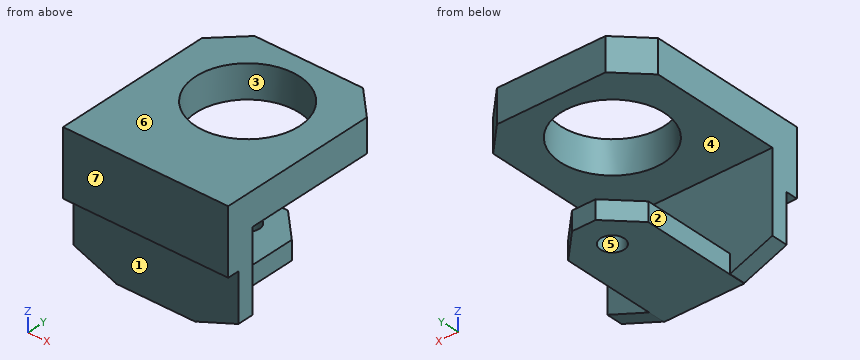
```python
from build123d import *

# Parameters (mm, degrees)
SKETCH1_W           = 35
SKETCH1_H           = 40
SKETCH1_R           = 11
BOSS_EXTRUDE1_DEPTH = 7
SKETCH2_W           = 35
SKETCH2_H           = 6
BOSS_EXTRUDE2_DEPTH = 16.5
SKETCH3_W           = 17
SKETCH3_H           = 32
SKETCH3_R           = 2.5
BOSS_EXTRUDE3_DEPTH = 4
CHAMFER1_SIZE       = 10.2
CHAMFER1_SIZE_2     = 3.915413157
CHAMFER2_SIZE       = 6
SKETCH4_W           = 35
SKETCH4_H           = 2.5
CUT_EXTRUDE1_DEPTH  = 13.7


with BuildPart() as part:
    # Sketch1 → Boss-Extrude1 (new body)
    with BuildSketch(Plane.XY):
        with Locations((0, -5)):
            Rectangle(SKETCH1_W, SKETCH1_H)
        Circle(SKETCH1_R, mode=Mode.SUBTRACT)
    extrude(amount=BOSS_EXTRUDE1_DEPTH)

    # Sketch2 → Boss-Extrude2 (add)
    with BuildSketch(Plane(origin=(0, 0, 0), x_dir=(-1, 0, 0), z_dir=(0, 0, -1))):
        with Locations((0, -22)):
            Rectangle(SKETCH2_W, SKETCH2_H)
    extrude(amount=BOSS_EXTRUDE2_DEPTH)

    # Sketch3 → Boss-Extrude3 (add)
    with BuildSketch(Plane(origin=(0, 0, -16.5), x_dir=(-1, 0, 0), z_dir=(0, 0, -1))):
        with Locations((0, -9)):
            Rectangle(SKETCH3_W, SKETCH3_H)
        Circle(SKETCH3_R, mode=Mode.SUBTRACT)
    extrude(amount=BOSS_EXTRUDE3_DEPTH)

    # Chamfer1
    # the kernel refuses this chamfer: 10.2, 3.915413157 mm, written as the material it adds along each edge
    with BuildSketch(Plane(origin=(-8.5, -19, -16.5), x_dir=(-0.9999045356599434, 0, 0.013817364679016049), z_dir=(0, -1, 0))) as chamfer1_piece_1_section:
        Polygon((CHAMFER1_SIZE * 0.99990453566, CHAMFER1_SIZE * 0.013817364679), (-CHAMFER1_SIZE_2 * 0.0138173646803, CHAMFER1_SIZE_2 * 0.999904535752), (0, 0), align=None)
    chamfer1_piece_1 = extrude(amount=6, mode=Mode.PRIVATE)
    chamfer1_piece_1 = split(chamfer1_piece_1, bisect_by=Plane(origin=(-17.5, -22, -17.821300415), z_dir=(1, 0, 0)), keep=Keep.TOP, mode=Mode.PRIVATE)
    add(chamfer1_piece_1)
    with BuildSketch(Plane(origin=(8.5, -25, -16.5), x_dir=(0.9999045356599434, 0, 0.013817364679016049), z_dir=(0, 1, 0))) as chamfer1_piece_2_section:
        Polygon((CHAMFER1_SIZE * 0.99990453566, CHAMFER1_SIZE * 0.013817364679), (-CHAMFER1_SIZE_2 * 0.0138173646803, CHAMFER1_SIZE_2 * 0.999904535752), (0, 0), align=None)
    chamfer1_piece_2 = extrude(amount=6, mode=Mode.PRIVATE)
    chamfer1_piece_2 = split(chamfer1_piece_2, bisect_by=Plane(origin=(17.5, -22, -17.821300415), z_dir=(-1, 0, 0)), keep=Keep.TOP, mode=Mode.PRIVATE)
    add(chamfer1_piece_2)

    # Chamfer2
    chamfer2_edges = [part.edges().sort_by_distance(p)[0] for p in [
        (-8.5, 7, -18.5),
        (8.5, 7, -18.5),
        (17.5, 15, 3.5),
        (-17.5, 15, 3.5),
    ]]
    chamfer(chamfer2_edges, length=CHAMFER2_SIZE)

    # Sketch4 → Cut-Extrude1 (cut)
    with BuildSketch(Plane(origin=(0, 0, -20.5), x_dir=(-1, 0, 0), z_dir=(0, 0, -1))):
        with Locations((0, -23.75)):
            Rectangle(SKETCH4_W, SKETCH4_H)
    extrude(amount=-CUT_EXTRUDE1_DEPTH, mode=Mode.SUBTRACT)


solid = part.part
```
Can you work these out from the model? Positions are in its coordinate system, mm. Face numbers are marked on the shaded views. A direction names the side the tool comes from. Give positions to 0.01 mm unless a question says otherwise; leave off trailing zeros. Loops run counter-clockwise (first coordinate to the right, second up) from the corner with the lowest first, then second, coordinate; pieces in that order, holes last. Notation, with made-up numbers: M 66,-25.75 L 111,-25.75 A33 ccw 111,9.25 Z; hole C -26.5,66.5 d5. An arc over 180 degrees is marked long. Use one line per item in the form item = value. Start each with the question number.
(1) I want a section at B-B, the plane y = -17.5. Write out the boundary of the cut face in (x, z), and give its area (3 significant figures).
(2) On a 3-axis mill with a long thin cutter (end or side, diameter ignored), from which of +Z, -Z, +X, -X, +Y, -Y can I reach the whole of each face in a straight line? I mean the marked faces 1, 2, 3 and 4. Say none if no direction works.
(3) I'm going to push flat-ended pins straight in: P1, Ø7, axis at x = -5.5, z = -14, coming from the -Y side; P2, Ø3, axis at x = -1.5, z = -16, coming from the +Y side; P3, Ø4.5, axis at y = -7, z = -18.5, coming from the -X side; P4, Ø1.5, axis at y = 0.5, z = -1.5, coming from the -X side. Where does each tip first touch, or does it pass through?
(4) Please list where these lines run through material, in increasing order: line 1 (Y direction, x = 0, z = 4); line 2 (Y direction, x = 0, z = -17.95); line 3 (Y direction, x = -4, z = -10.75).
(5) Thinking about a two-plate mould opening in Y: for the marked faces 5, 6 and 7, which applies, released by +Y, released by -Y, zero draft, split by the parting line, or undercut?
(6) I want a section at C-C, the plane y = 0. Write out the boundary of the cut face in (x, z).
(7) I want a section at D-D, the plane z = 5.25. Write out the boundary of the cut face in (x, y).
(8) I want a section at A-A, the plane x = 0. Write out the boundary of the cut face in (y, z).
Worked out:
q1.outline = M -17.5,0 L 17.5,0 L 17.5,7 L -17.5,7 Z; M -8.5,-20.5 L 8.5,-20.5 L 8.5,-16.5 L -8.5,-16.5 Z
q1.area = 313 mm²
q2.face_1 = -Z, +X, -X, -Y
q2.face_2 = -Z, -X, +Y
q2.face_3 = +Z
q2.face_4 = +X, -X, +Y
q3.P1 = -22.5
q3.P2 = 7
q3.P3 = -8.5
q3.P4 = through
q4.line_1 = -25 to -11, 11 to 15
q4.line_2 = -22.5 to -2.5, 2.5 to 7
q4.line_3 = -22.5 to -19
q5.face_5 = undercut
q5.face_6 = zero draft
q5.face_7 = released by -Y
q6.outline = M -17.5,0 L -11,0 L -11,7 L -17.5,7 Z; M -8.5,-20.5 L -2.5,-20.5 L -2.5,-16.5 L -8.5,-16.5 Z; M 2.5,-20.5 L 8.5,-20.5 L 8.5,-16.5 L 2.5,-16.5 Z; M 11,0 L 17.5,0 L 17.5,7 L 11,7 Z
q7.outline = M -17.5,-25 L 17.5,-25 L 17.5,9 L 11.5,15 L -11.5,15 L -17.5,9 Z; hole C 0,0 d22
q8.outline = M -25,-6.8 L -22.5,-6.8 L -22.5,-20.5 L -2.5,-20.5 L -2.5,-16.5 L -19,-16.5 L -19,0 L -11,0 L -11,7 L -25,7 Z; M 2.5,-20.5 L 7,-20.5 L 7,-16.5 L 2.5,-16.5 Z; M 11,0 L 15,0 L 15,7 L 11,7 Z
